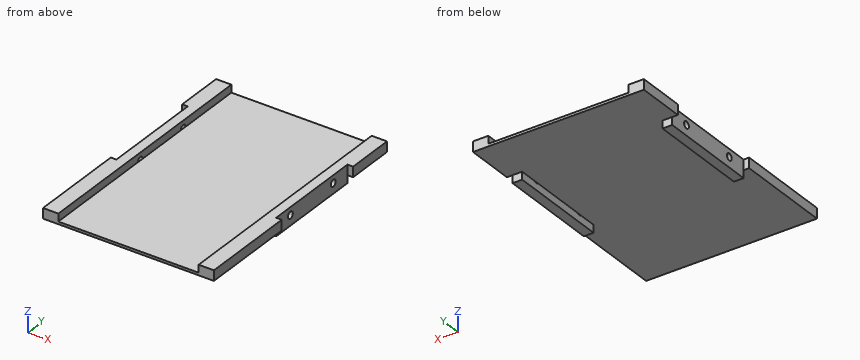
Autodesk Inventor part; units mm, degrees
ref_plane "YZ Plane" through (0, 0, 0) normal (1, 0, 0) x (0, 1, 0)
ref_plane "XZ Plane" through (0, 0, 0) normal (0, 1, 0) x (-1, 0, 0)
ref_plane "XY Plane" through (0, 0, 0) normal (0, 0, 1) x (1, 0, 0)
sketch "スケッチ1" plane through (0, 0, 0) normal (0, 0, 1) x (1, 0, 0)
  line L0 (33.5, -48.5) -> (-33.5, -48.5)
  line L1 (-33.5, -48.5) -> (-33.5, 48.5)
  line L2 (-33.5, 48.5) -> (33.5, 48.5)
  line L3 (33.5, 48.5) -> (33.5, -48.5)
  line L4 (33.5, -48.5) -> (-33.5, 48.5) construction
  line L5 (-33.5, -48.5) -> (33.5, 48.5) construction
  point P0 (0, 0)
  dimension "d0" = 67
  dimension "d1" = 97
extrude "押し出し1" add sketch "スケッチ1" along normal blind 1
sketch "スケッチ3" plane through (33.5, -48.5, 0) normal (1, 0, 0) x (0, 0, -1)
  line L0 (0, 78) -> (-5, 78)
  line L1 (-5, 78) -> (-5, 38)
  line L2 (-5, 38) -> (0, 38)
  line L3 (0, 38) -> (0, 78)
  circle A0 centre (-1, 70) radius 1.35
  line L4 (0, 97) -> (-1, 97)
  line L5 (0, 0) -> (0, 97)
  circle A1 centre (-1, 46) radius 1.35
  point P0 (0, 48.5)
  dimension "d4" = 5
  dimension "d5" = 27
  dimension "d6" = 8
  dimension "d7" = 40
  dimension "d8" = 2.7
  dimension "d9" = 8
  dimension "d48" = 1
extrude "押し出し2" add sketch "スケッチ3" against normal blind 6 contours L3 A0 A1 L2 L1 L0
extrude "押し出し3" cut sketch "スケッチ3" against normal blind 2.2 contours L3 A0 A1 L2 L1 L0
mirror "ミラー1" about plane through (0, 0, 0) normal (1, 0, 0) of "押し出し2", "押し出し3"
sketch "スケッチ12" plane through (31.3, -48.5, 0) normal (1, 0, 0) x (0, 0, -1)
  line L0 (-1, 78) -> (-5, 78)
  line L1 (-5, 78) -> (3, 78)
  line L2 (3, 78) -> (3, 38)
  line L3 (3, 38) -> (-5, 38)
  line L4 (-5, 38) -> (-5, 78)
  arc A0 (-1, 71.35) -> (-1, 68.65) centre (-1, 70) ccw
  arc A1 (-1, 47.35) -> (-1, 44.65) centre (-1, 46) ccw
  circle A2 centre (-1, 70) radius 1.35
  circle A3 centre (-1, 46) radius 1.35
  point P0 (0, 48.5)
  point P1 (0, 38)
  point P2 (-1, 68.65)
  point P3 (-1, 44.65)
  dimension "d49" = 8
extrude "押し出し15" add sketch "スケッチ12" against normal up to surface (3.8 mm away)
sketch "スケッチ13" plane through (27.5, -10.5, -3) normal (-1, 0, 0) x (0, 0, 1)
  line L0 (4, 30.65) -> (4, 33.35)
  circle A0 centre (4, 32) radius 1.35
  line L1 (4, 6.65) -> (4, 9.35)
  circle A1 centre (4, 8) radius 1.35
  arc A2 (4, 30.65) -> (4, 33.35) centre (4, 32) ccw
  arc A3 (4, 6.65) -> (4, 9.35) centre (4, 8) ccw
  point P0 (3, 10.5)
extrude "押し出し16" cut sketch "スケッチ13" against normal through all
mirror "ミラー2" about plane through (0, 0, 0) normal (1, 0, 0) of "押し出し15", "押し出し16"
sketch "スケッチ14" plane through (0, 0, 1) normal (0, 0, 1) x (1, 0, 0)
  line L0 (-27.5, -10.5) -> (-27.5, 29.5)
  line L1 (27.5, -10.5) -> (27.5, 29.5)
  line L2 (33.5, 48.5) -> (-33.5, 48.5)
  line L3 (-33.5, -48.5) -> (33.5, -48.5)
  line L4 (-27.5, 48.5) -> (27.5, 48.5)
  line L5 (27.5, 48.5) -> (27.5, -48.5)
  line L6 (27.5, -48.5) -> (-27.5, -48.5)
  line L7 (-27.5, -48.5) -> (-27.5, 48.5)
  line L8 (-27.5, 22.85) -> (-27.5, 20.15)
  line L9 (-27.5, 20.15) -> (-27.5, -1.15)
  line L10 (-27.5, -1.15) -> (-27.5, -3.85)
  line L11 (-27.5, -3.85) -> (-27.5, -10.5)
  line L12 (-27.5, -10.5) -> (-31.3, -10.5)
  line L13 (-31.3, -10.5) -> (-33.5, -10.5)
  line L14 (-33.5, -10.5) -> (-33.5, -48.5)
  line L15 (-33.5, -48.5) -> (33.5, -48.5)
  line L16 (33.5, -48.5) -> (33.5, -10.5)
  line L17 (33.5, -10.5) -> (31.3, -10.5)
  line L18 (31.3, -10.5) -> (27.5, -10.5)
  line L19 (27.5, -10.5) -> (27.5, -3.85)
  line L20 (27.5, -3.85) -> (27.5, -1.15)
  line L21 (27.5, -1.15) -> (27.5, 20.15)
  line L22 (27.5, 20.15) -> (27.5, 22.85)
  line L23 (27.5, 22.85) -> (27.5, 29.5)
  line L24 (27.5, 29.5) -> (31.3, 29.5)
  line L25 (31.3, 29.5) -> (33.5, 29.5)
  line L26 (33.5, 29.5) -> (33.5, 48.5)
  line L27 (33.5, 48.5) -> (-33.5, 48.5)
  line L28 (-33.5, 48.5) -> (-33.5, 29.5)
  line L29 (-33.5, 29.5) -> (-31.3, 29.5)
  line L30 (-31.3, 29.5) -> (-27.5, 29.5)
  line L31 (-27.5, 29.5) -> (-27.5, 22.85)
  point P0 (0, 0)
  point P1 (-27.5, -48.5)
extrude "押し出し17" add sketch "スケッチ14" along normal up to surface (4 mm away) contours L7 L3 L14 L13 L12 | L5 L18 L17 L16 L3 | L30 L29 L28 L2 L7 | L2 L26 L25 L24 L5
sketch "スケッチ15" plane through (-33.5, -48.5, 5) normal (0, 0, 1) x (1, 0, 0)
  line L0 (2.2, 78) -> (2.2, 38)
  line L1 (0, 38) -> (2.2, 38)
  line L2 (0, 0) -> (0, 38)
  line L3 (6, 0) -> (0, 0)
  line L4 (6, 97) -> (6, 0)
  line L5 (0, 97) -> (6, 97)
  line L6 (0, 78) -> (0, 97)
  line L7 (2.2, 78) -> (0, 78)
  line L8 (64.8, 38) -> (64.8, 78)
  line L9 (67, 78) -> (64.8, 78)
  line L10 (67, 97) -> (67, 78)
  line L11 (61, 97) -> (67, 97)
  line L12 (61, 0) -> (61, 97)
  line L13 (67, 0) -> (61, 0)
  line L14 (67, 38) -> (67, 0)
  line L15 (64.8, 38) -> (67, 38)
  point P0 (33.5, 48.5)
extrude "押し出し18" cut sketch "スケッチ15" against normal blind 1
equation "\"d9\" = d6"
equation "\"BendRadius\" = Thickness"
equation "\"BendReliefWidth\" = Thickness"
equation "\"BendReliefDepth\" = 0.5 * Thickness"
equation "\"CornerReliefSize\" = 4 * Thickness"
equation "\"MinimumRemnant\" = 2 * Thickness"
equation "\"TransitionRadius\" = BendRadius"
equation "\"JacobiRadiusSize\" = BendRadius"
equation "\"GapSize\" = Thickness"
properties part number "cover_right"
Here's how the part is built. I have some questions about the finished solid (model axes, mm). Give positions to 0.01 mm unless a question says otherwise; leave off trailing zeros. Order: outer loops, then holes, each group sorted by start corner. A loop starts at its lowest first (then second) coordinate and runs counter-clockwise, first axis right, second up. Notation, with made-up numbers: (51, -30.75) -> (76, -30.75) arc R31 cw to (76, -2.75) -> close; hole circle Ø8 at (24.5, 41). An arc over 180 degrees is marked (long way). One line per item, written item: value. Start each with the question number.
1. Imagine slicing it at C-C, the plane x = -11. List the corners of the cut face in (y, z) for me.
2. Imagine slicing it at B-B, the plane y = 11. List the corners of the cut face in (x, z) for me.
3. Imagine slicing it at D-D, the plane y = 36. List the corners of the cut face in (x, z) for me, plus the area to 3 significant figures.
4. Imagine slicing it at A-A, the plane z = -2. List the corners of the cut face in (x, y) for me, plus the area to 3 significant figures.
5. Will these pins go through, and if not, where does the flat tip stop? pin 1 Ø12 at (x, y) = (-3.5, -13) entering from -Z; pin 2 Ø1.5 at (y, z) = (12.5, -2) entering from +X; pin 3 Ø1.5 at (y, z) = (-1.5, 0.5) entering from -X; pin 4 Ø1 at (x, z) = (-11, 2.5) entering from -Y.
6. I need wall thicknesses on probe 1 along Y at (x, z) = (-29.95, 1); probe 2 along Z at (x, y) = (-28.8, -2.5); probe 3 along X at (y, z) = (9, -2.5). Which ranges of each line are inside material? Lowest first, please. Write a range as from..to.
Values follow:
1. outline: (-48.5, 0) -> (48.5, 0) -> (48.5, 1) -> (-48.5, 1) -> close
2. outline: (-31.3, -3) -> (-27.5, -3) -> (-27.5, 0) -> (27.5, 0) -> (27.5, -3) -> (31.3, -3) -> (31.3, 4) -> (27.5, 4) -> (27.5, 1) -> (-27.5, 1) -> (-27.5, 4) -> (-31.3, 4) -> close
3. outline: (-33.5, 0) -> (33.5, 0) -> (33.5, 4) -> (27.5, 4) -> (27.5, 1) -> (-27.5, 1) -> (-27.5, 4) -> (-33.5, 4) -> close
3. area: 103 mm2
4. outline: (-31.3, -10.5) -> (-27.5, -10.5) -> (-27.5, 29.5) -> (-31.3, 29.5) -> close; (27.5, -10.5) -> (31.3, -10.5) -> (31.3, 29.5) -> (27.5, 29.5) -> close
4. area: 304 mm2
5. pin 1: stops at z = 0
5. pin 2: stops at x = 31.3
5. pin 3: stops at x = -31.3
5. pin 4: passes through
6. probe 1: y = -48.5..-3.85, -1.15..20.15, 22.85..48.5
6. probe 2: z = -3..-0.35, 2.35..4
6. probe 3: x = -31.3..-27.5, 27.5..31.3
